Autodesk Inventor part; units mm, degrees
ref_plane "YZ Plane" through (0, 0, 0) normal (1, 0, 0) x (0, 1, 0)
ref_plane "XZ Plane" through (0, 0, 0) normal (0, 1, 0) x (-1, 0, 0)
ref_plane "XY Plane" through (0, 0, 0) normal (0, 0, 1) x (1, 0, 0)
sketch "草图1" plane through (0, 0, 0) normal (0, 0, 1) x (1, 0, 0)
  circle A0 centre (0, 0) radius 7.5
  dimension "d0" = 15
extrude "拉伸1" add sketch "草图1" along normal blind 5
sketch "草图2" plane through (0, 0, 5) normal (0, 0, 1) x (1, 0, 0)
  circle A0 centre (0, 0) radius 5
  dimension "d3" = 10
extrude "拉伸2" add sketch "草图2" along normal blind 490
sketch "草图3" plane through (0, 0, 0) normal (0, 1, 0) x (-1, 0, 0)
  circle A0 centre (0, 493) radius 1
  line L0 (5, 495) -> (-5, 495)
  point P0 (0, 0)
  dimension "d6" = 2
  dimension "d7" = 2
extrude "拉伸3" cut sketch "草图3" along normal through all both and the other way through all
sketch "草图4" plane through (0, 0, 495) normal (0, 0, 1) x (1, 0, 0)
  circle A0 centre (0, 0) radius 4
  circle A1 centre (0, 0) radius 5
  dimension "d15" = 8
  dimension "d16" = 10
extrude "拉伸4" cut sketch "草图4" against normal blind 7
thread "螺纹2"
chamfer "倒角2" distance 0.25 angle 45 1 edges at (-4, 0, 495)
properties part number "砂轮架固定销"
CAD build for the part. Positions are in the model's coordinates, mm. A direction names the side the tool comes from. Coordinates: 2 decimals unless noted, no trailing zeros. Loops run counter-clockwise (first coordinate to the right, second up) from the corner with the lowest first, then second, coordinate; pieces in that order, holes last. Notation, with made-up numbers: (-21.5, 31) - (-3.5, 31) arc R13 cw to (-3.5, 40) - close; hole circle Ø11 at (-16, 4.25). An arc over 180 degrees is marked (long way). Use CSV: the item, a comma, the result in double quotes. Start each with the question number.
Q1. Drop flat-ended pins along their axis: P1, Ø4, axis at x = -0.5, z = 417.5, coming from the +Y side; P2, Ø8, axis at y = 4.5, z = 203, coming from the -X side; P3, Ø5, axis at x = 5, z = 311, coming from the +Y side. Give the stop position or say it passes through.
Q2. Cut at B-B, the plane z = 380. List the corners of the cut face in (x, y), then the cut area to 3 significant figures.
Q3. Cut at A-A, the plane y = 0. List the corners of the cut face in (x, z), then the cut area to 3 significant figures.
Q4. Probe probe 1 along X at (y, z) = (0.5, 493); probe 2 along Z at (x, y) = (0, 0.75); probe 3 along X at (y, z) = (-1.5, 493). List the from-to ranges inside material, lowest first. Write a range as from..to.
Q5. 3-axis set-ups, long thin cutter, end or side, ignore diameter. For faces 1 (the cylindrical face through (-7.493, -0.33, 2.465)), 2 (the flat face through (2, -5, 5)): which of +Z, -Z, +X, -X, +Y, -Y reach the whole face in a straight line?
Here are the results:
1,P1,"y = 5"
1,P2,"x = -4.97"
1,P3,"y = 4.33"
2,outline,"circle Ø10 at (0, 0)"
2,area,"78.5 mm2"
3,outline,"(-7.5, 0) - (7.5, 0) - (7.5, 5) - (5, 5) - (5, 488) - (4, 488) - (4, 494.75) - (3.75, 495) - (-3.75, 495) - (-4, 494.75) - (-4, 488) - (-5, 488) - (-5, 5) - (-7.5, 5) - close; hole circle Ø2 at (0, 493)"
3,area,"4,960 mm2"
4,probe 1,"-3.97..-1, 1..3.97"
4,probe 2,"0..492, 494..495"
4,probe 3,"-3.71..-1, 1..3.71"
5,face 1,"+Z, -Z"
5,face 2,"+Z"
